Check sheet for the modelled part. Datum: model origin and axes. Units: mm. A direction names the side the tool comes from. Give positions to 0.01 mm unless a question says otherwise; leave off trailing zeros. Write each loop counter-clockwise with the first axis right and the second up, starting at its lowest first coordinate (ties: lowest second). Pieces come first, ordered by that corner, then holes. Notation, with made-up numbers: M 36,58 L 67,58 A12 ccw 67,74 Z; hole C -13.5,58.25 d1. An arc over 180 degrees is marked long. Use CSV: the item, a comma, the result in double quotes. Start each with the question number.
1. Access from +Z, -Z, +X, -X, +Y, -Y to the whole of each face (thin tool, end or side, straight path). Record for faces 1 (the face through (44.5, 5, -108)), 2 (the face through (0, -23, -110.625)), 3 (the face through (34, -25.656, -108)).
2. Cross-section at D-D, the plane y = 54.5. Enter the section's corners in (x, z) (3 decimals), and give its area (3 significant figures).
3. Cross-section at A-A, the plane y = 0. Enter the section's corners in (x, z) (3 decimals), and give its area (3 significant figures).
4. Mould release check, pull along Y, two halves, no side actions. Record for faces 4 (the face through (-44.5, 5, -108)), 5 (the face through (0.547, -60.629, -107.945)), 6 (the face through (0, -23, -105.189)): +Y half, -Y half, draft (parallel to the pull), parting line (faces both ways), or undercut.
5. Scan lines: line 1 (X direction, y = -10, z = -108.85); line 2 (Y direction, x = -20, z = -108.45); line 3 (X direction, y = 45, z = -108.15). Record each from-to range of solid material in increasing order.
6. Cross-section at B-B, the plane x = 11. Enter the section's corners in (y, z) (3 decimals).
7. Depth check by flat-ended pin: P1, Ø5, axis at x = 51.25, y = 23.18, coming from the -Z side; P2, Ø7, axis at x = -51.25, y = -12.5, coming from the +Z side; P3, Ø1.6, axis at y = 4.5, z = -107, coming from the -X side; P4, Ø2.5, axis at x = -12.5, z = -107, coming from the +Y side. Enter the tip coordinate at first touch or a pass-through.
8. Cross-section at C-C, the plane z = -109.15. State how many separate pieces and enclosed holes the cut face has, and give its area (3 significant figures).
from build123d import *

# Parameters (mm, degrees)
SKETCH2_R           = 10
SKETCH2_R_2         = 2.75
SKETCH2_R_3         = 1.25
SKETCH2_W           = 89
SKETCH2_H           = 52
BOSS_EXTRUDE1_DEPTH = 5.4356


with BuildPart() as part:
    # Sketch2 → Boss-Extrude1 (new body)
    with BuildSketch(Plane(origin=(0, 0, -110.625), x_dir=(-1, 0, 0), z_dir=(0, 0, -1))):
        with BuildLine():
            Line((-4.357448371, -54.013133709), (-6.946028661, -34.350914325))
            ThreePointArc((-6.946028661, -34.350914325), (-10.267019124, -28.137778173), (-16.860477275, -25.656176248))
            Line((-16.860477275, -25.656176248), (-50.634811595, -25.656176248))
            ThreePointArc((-50.634811595, -25.656176248), (-56.570299984, -23.704155969), (-60.188549632, -18.610171766))
            ThreePointArc((-60.188549632, -18.610171766), (34.680301225, 52.595405759), (6.605490855, -62.652753256))
            ThreePointArc((6.605490855, -62.652753256), (-0.632673359, -60.562038878), (-4.357448371, -54.013133709))
        make_face()
        with Locations(Location((12.5, 46.343823752, 0), (0, 0, 90))):
            Circle(SKETCH2_R, mode=Mode.SUBTRACT)
        with Locations(Location((-12.5, 46.343823752, 0), (0, 0, 90))):
            Circle(SKETCH2_R, mode=Mode.SUBTRACT)
        with Locations(Location((32.134671235, -35.656176248, 0), (0, 0, 90))):
            Circle(SKETCH2_R, mode=Mode.SUBTRACT)
        with Locations(Location((9.845967479, -46.979324435, 0), (0, 0, 90))):
            Circle(SKETCH2_R, mode=Mode.SUBTRACT)
        with Locations(Location((51.25, 23.184046239, 0), (0, 0, 90))):
            Circle(SKETCH2_R_2, mode=Mode.SUBTRACT)
        with Locations(Location((51.25, -12.496398734, 0), (0, 0, 90))):
            Circle(SKETCH2_R_2, mode=Mode.SUBTRACT)
        with Locations(Location((-51.25, -12.496398734, 0), (0, 0, 90))):
            Circle(SKETCH2_R_2, mode=Mode.SUBTRACT)
        with Locations(Location((-51.25, 23.184046239, 0), (0, 0, 90))):
            Circle(SKETCH2_R_2, mode=Mode.SUBTRACT)
        with Locations(Location((13.291416771, -25.156176248, 0), (0, 0, 90))):
            Circle(SKETCH2_R_3, mode=Mode.SUBTRACT)
        with Locations(Location((-0.708583229, -25.156176248, 0), (0, 0, 90))):
            Circle(SKETCH2_R_3, mode=Mode.SUBTRACT)
        with Locations((0, 5.343823752)):
            Rectangle(SKETCH2_W, SKETCH2_H, mode=Mode.SUBTRACT)
    extrude(amount=-BOSS_EXTRUDE1_DEPTH)


solid = part.part
Worked answers:
1,face 1,"+Z, -Z"
1,face 2,"-Z, +X, -X, +Y, -Y"
1,face 3,"+Z, -Z, +X, -Y"
2,outline,"M -31.603,-110.625 L -18.286,-110.625 L -18.286,-105.189 L -31.603,-105.189 Z; M -6.714,-110.625 L 6.714,-110.625 L 6.714,-105.189 L -6.714,-105.189 Z; M 18.286,-110.625 L 31.603,-110.625 L 31.603,-105.189 L 18.286,-105.189 Z"
2,area,"218 mm^2"
3,outline,"M -63,-110.625 L -44.5,-110.625 L -44.5,-105.189 L -63,-105.189 Z; M 44.5,-110.625 L 63,-110.625 L 63,-105.189 L 44.5,-105.189 Z"
3,area,"201 mm^2"
4,face 4,"undercut"
4,face 5,"-Y half"
4,face 6,"draft"
5,line 1,"x = -62.2 to -52.4, -50.1 to -44.5, 44.5 to 50.1, 52.4 to 62.2"
5,line 2,"y = -59.74 to -20.66, 31.34 to 39.73, 52.96 to 59.74"
5,line 3,"x = -44.09 to -22.41, -2.59 to 2.59, 22.41 to 44.09"
6,outline,"M -27.553,-110.625 L -20.656,-110.625 L -20.656,-105.189 L -27.553,-105.189 Z; M 31.344,-110.625 L 36.457,-110.625 L 36.457,-105.189 L 31.344,-105.189 Z; M 56.231,-110.625 L 62.032,-110.625 L 62.032,-105.189 L 56.231,-105.189 Z"
7,P1,"passes through"
7,P2,"stops at z = -105.19"
7,P3,"stops at x = -62.89"
7,P4,"stops at y = 61.99"
8,separate pieces,"1"
8,enclosed holes,"11"
8,area,"5,130 mm^2"
